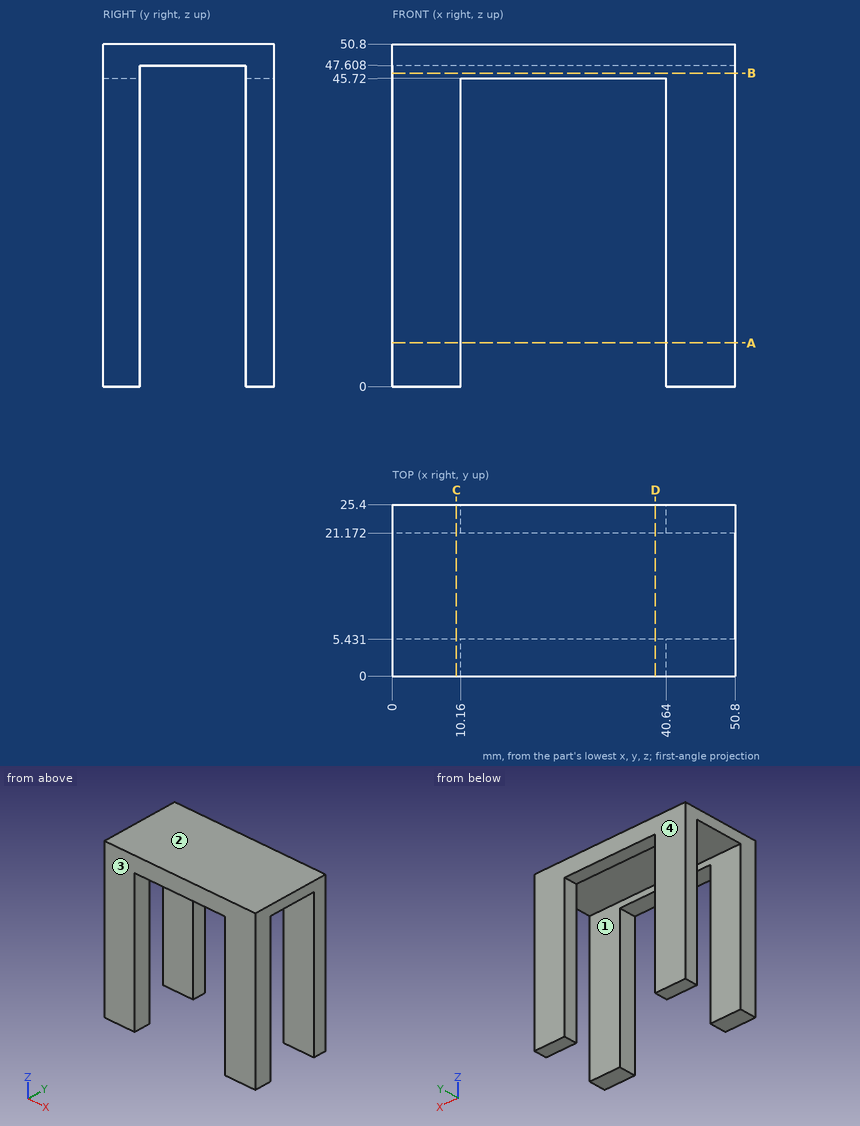
The figure shows three views and two pictorial views of one solid part (mm, origin at its lowest corner). Answer the questions. Round coordinates to 2 decimals unless told otherwise and drop trailing zeros. Loops run counter-clockwise (first coordinate to the right, second up) from the corner with the lowest first, then second, coordinate; pieces in that order, holes last. Notation, with made-up numbers: M -26.5,-25.5 L 6.5,-25.5 A38 ccw 6.5,12.5 Z; hole C 59,64 d3. An arc over 180 degrees is marked long. Return JSON: item names as keys, results as strings.
Q1. Find section B-B, the plane z = 46.5. Determine the outline of the cut face in (x, y).
Results list:
{"outline": "M 0,0 L 50.8,0 L 50.8,5.43 L 0,5.43 Z; M 0,21.17 L 50.8,21.17 L 50.8,25.4 L 0,25.4 Z"}
Q2. Find section A-A, the plane z = 6.5. Determine the outline of the cut face in (x, y).
Results list:
{"outline": "M 0,0 L 10.16,0 L 10.16,5.43 L 0,5.43 Z; M 0,21.17 L 10.16,21.17 L 10.16,25.4 L 0,25.4 Z; M 40.64,0 L 50.8,0 L 50.8,5.43 L 40.64,5.43 Z; M 40.64,21.17 L 50.8,21.17 L 50.8,25.4 L 40.64,25.4 Z"}
Q3. Find the intervals of material crossed by line 1 along Y through (x, z) = (27.5, 47.5); line 2 along X through (y, z) = (2.5, 14.5); line 3 along Z through (x, y) = (2, 19), in increasing order. Write a range as from..to.
Results list:
{"line 1": "y = 0..5.43, 21.17..25.4", "line 2": "x = 0..10.16, 40.64..50.8", "line 3": "z = 47.61..50.8"}
Q4. Find section D-D, the plane x = 39. Determine the outline of the cut face in (y, z), plus the area to 3 significant figures.
Results list:
{"outline": "M 0,45.72 L 5.43,45.72 L 5.43,47.61 L 21.17,47.61 L 21.17,45.72 L 25.4,45.72 L 25.4,50.8 L 0,50.8 Z", "area": "99.3 mm2"}
Q5. Find section C-C, the plane x = 9.5. Determine the outline of the cut face in (y, z).
Results list:
{"outline": "M 0,0 L 5.43,0 L 5.43,47.61 L 21.17,47.61 L 21.17,0 L 25.4,0 L 25.4,50.8 L 0,50.8 Z"}
Q6. Each of these flat-tipped pins is pushed along its axis until it touches: pin 1 Ø1.6 at (x, y) = (27, 4) entering from -Z; pin 2 Ø14.5 at (x, z) = (28.5, 35.5) entering from +Y; pin 3 Ø8 at (x, y) = (29.5, 13) entering from -Z. Where does it stop, or does it pass through?
Results list:
{"pin 1": "stops at z = 45.72", "pin 2": "passes through", "pin 3": "stops at z = 47.61"}
Q7. The mould has two halves that part along Y. Classify the marked faces 1, 2, 3 and 4: released by +Y, released by -Y, zero draft, split by the parting line, or undercut.
Results list:
{"face 1": "undercut", "face 2": "zero draft", "face 3": "released by -Y", "face 4": "released by +Y"}
